Answer from the drawing. Dimensions are ordinates in mm from the lowest x, y and z of the part. Coordinates: 2 decimals unless noted, no trailing zeros. Write each loop counter-clockwise with the first axis right and the second up, starting at its lowest first coordinate (ties: lowest second). Pieces come first, ordered by that corner, then holes.
(1) The mould has two halves that part along X. Classify the marked faces 1, 2 and 3: +X half, -X half, draft (parallel to the pull), parting line (faces both ways), or undercut.
(2) Find the intervals of material crossed by probe 1 along X at (y, z) = (5, 3.75) (1 decimal); probe 2 along Y at (x, z) = (4, 3.25) (1 decimal); probe 3 along Z at (x, y) = (4, 9) (1 decimal), in increasing order.
(3) Given pin 1 (1.5 mm diameter, centred on x = 3, z = 4.5, fed in from +Y); pin 2 (3 mm diameter, centred on y = 7.5, z = 7, fed in from -X); pin 3 (5 mm diameter, centred on x = 2.5, y = 6.5, fed in from -Z); pin 4 (2 mm diameter, centred on x = 4, z = 6.5, fed in from +Y), each flat-ended and moving along its own axis, determine where each tip first touches the part or whether it passes through.
(4) Section A-A on y = 4 is taken. Write down the section's boundary in (x, z) (1 decimal).
(5) Section C-C on y = 7.25 is taken. Write down the section's boundary in (x, z) (1 decimal).
(6) Section D-D on x = 3 is taken. Write down the section's boundary in (y, z) (1 decimal).
(7) Section B-B on x = 5.25 is taken. Write down the section's boundary in (y, z) (1 decimal).
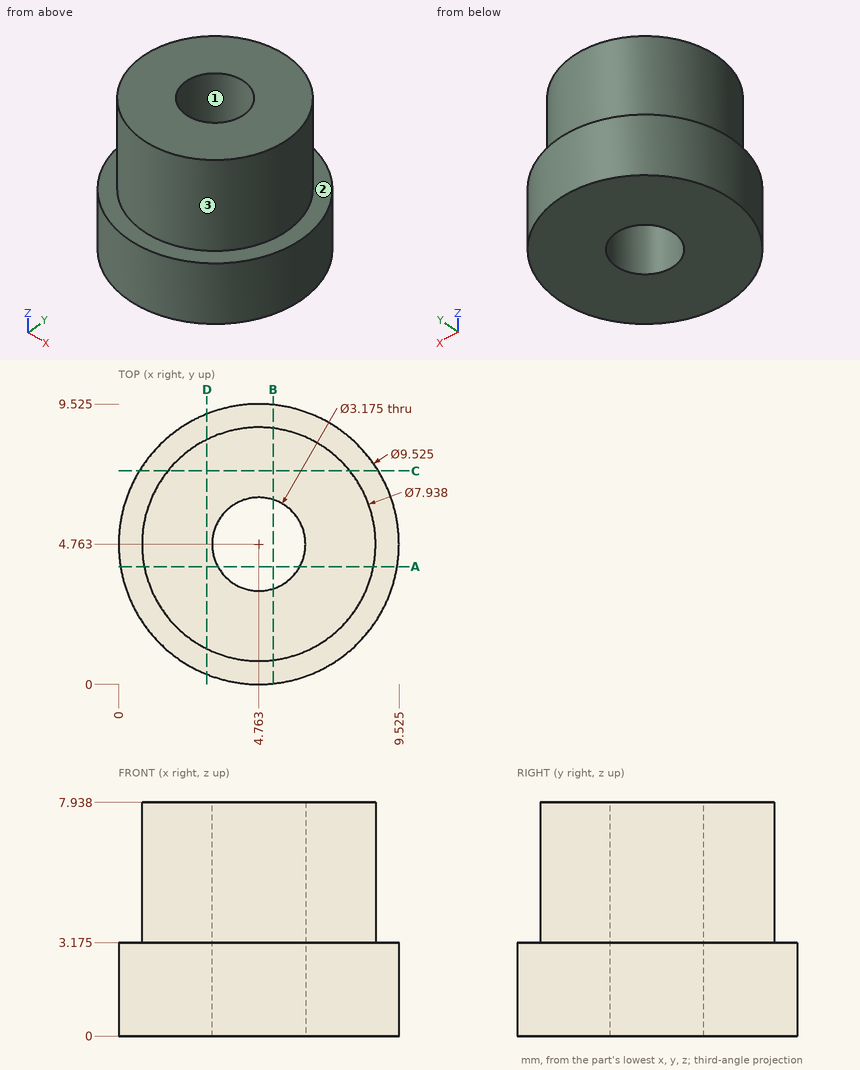
Response:
1. face 1: undercut
1. face 2: draft
1. face 3: parting line
2. probe 1: x = 0.8 to 3.2, 6.3 to 8.7
2. probe 2: y = 0.9 to 3.4, 6.2 to 8.7
2. probe 3: z = 0 to 3.2
3. pin 1: stops at y = 8.6
3. pin 2: stops at x = 0.99
3. pin 3: stops at z = 0
3. pin 4: stops at y = 8.73
4. outline: (0.1, 0) - (3.4, 0) - (3.4, 7.9) - (0.9, 7.9) - (0.9, 3.2) - (0.1, 3.2) - close; (6.2, 0) - (9.5, 0) - (9.5, 3.2) - (8.7, 3.2) - (8.7, 7.9) - (6.2, 7.9) - close
5. outline: (0.7, 0) - (8.8, 0) - (8.8, 3.2) - (7.9, 3.2) - (7.9, 7.9) - (1.7, 7.9) - (1.7, 3.2) - (0.7, 3.2) - close
6. outline: (0.3, 0) - (9.2, 0) - (9.2, 3.2) - (8.3, 3.2) - (8.3, 7.9) - (1.2, 7.9) - (1.2, 3.2) - (0.3, 3.2) - close
7. outline: (0, 0) - (3.3, 0) - (3.3, 7.9) - (0.8, 7.9) - (0.8, 3.2) - (0, 3.2) - close; (6.3, 0) - (9.5, 0) - (9.5, 3.2) - (8.7, 3.2) - (8.7, 7.9) - (6.3, 7.9) - close
